```python
from build123d import *

# Parameters (mm, degrees)
SKETCH1_R           = 1.25
BOSS_EXTRUDE1_DEPTH = 1.5
SKETCH3_W           = 18.5
SKETCH3_H           = 10
BOSS_EXTRUDE2_DEPTH = 2.53


with BuildPart() as part:
    # Sketch1 → Boss-Extrude1 (new body)
    with BuildSketch(Plane(origin=(0, 0, 0), x_dir=(1, 0, 0), z_dir=(0, 1, 0))):
        with BuildLine():
            Line((31.88, 2.5), (31.88, 18.9))
            ThreePointArc((31.88, 18.9), (31.147766953, 20.667766953), (29.38, 21.4))
            Line((29.38, 21.4), (0, 21.4))
            Line((0, 21.4), (0, 0))
            Line((0, 0), (29.38, 0))
            ThreePointArc((29.38, 0), (31.147766953, 0.732233047), (31.88, 2.5))
        make_face()
        with Locations((29.38, 2.5)):
            Circle(SKETCH1_R, mode=Mode.SUBTRACT)
        with Locations((29.38, 18.9)):
            Circle(SKETCH1_R, mode=Mode.SUBTRACT)
    extrude(amount=BOSS_EXTRUDE1_DEPTH)

    # Sketch3 → Boss-Extrude2 (add)
    with BuildSketch(Plane(origin=(0, 1.5, 0), x_dir=(1, 0, 0), z_dir=(0, 1, 0))):
        with Locations((22.63, 10.7)):
            Rectangle(SKETCH3_W, SKETCH3_H)
    extrude(amount=BOSS_EXTRUDE2_DEPTH)


solid = part.part
```
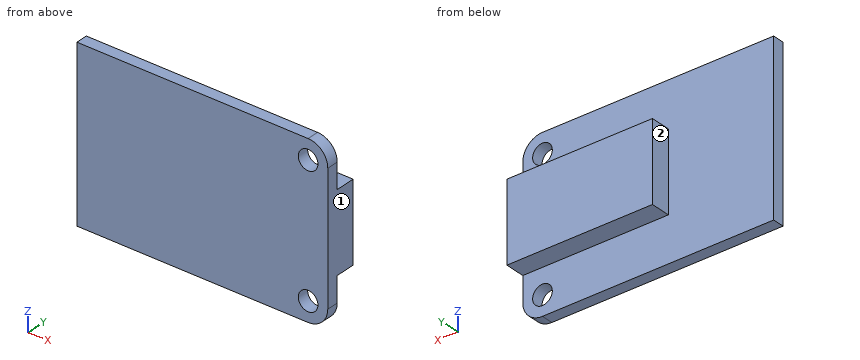
Geometry: final body of the model. Coordinates: model frame, mm. Face numbers are marked on the shaded views. A direction names the side the tool comes from. Give positions to 0.01 mm unless a question says otherwise; leave off trailing zeros. Order: outer loops, then holes, each group sorted by start corner. A loop starts at its lowest first (then second) coordinate and runs counter-clockwise, first axis right, second up. Notation, with made-up numbers: M -15.75,28.25 L -7.75,28.25 A13 ccw -7.75,50.25 Z; hole C 66,5 d4. An arc over 180 degrees is marked long. Answer as CSV lines item,"result". Start each with the question number.
1) Set-up query: the marked faces 1 and 2. Return all of +Z, -Z, +X, -X, +Y, -Y with unobstructed straight access to the full face (end or side cutting, diameter ignored); none if empty.
2) Cut plane A-A (x = 27). Output: boundary loops of the cut face in (y, z).
3) Cut plane C-C (y = 2.8). Output: boundary loops of the cut face in (x, z).
4) Cut plane D-D (x = 8). Output: boundary loops of the cut face in (y, z).
5) First-contact query: P1, Ø6, axis at x = 10, z = -10.5, coming from the -Y side; P2, Ø1.5, axis at x = 29.38, z = -18.9, coming from the +Y side. Flat tips, straight axial feed; report the tip coordinate or a pass-through.
6) Line query: line 1 (Z direction, x = 29.38, y = 1); line 2 (X direction, y = 1.05, z = -18.9); line 3 (X direction, y = 2.4, z = -14.5). Output: solid intervals per line, ascending. Write a range as from..to.
7) Cut plane B-B (z = -14.75). Output: boundary loops of the cut face in (x, y).
Findings below:
1,face 1,"+Z, -Z, +X, +Y, -Y"
1,face 2,"+Z, -Z, -X, +Y"
2,outline,"M 0,-21.4 L 1.5,-21.4 L 1.5,-15.7 L 4.03,-15.7 L 4.03,-5.7 L 1.5,-5.7 L 1.5,0 L 0,0 Z"
3,outline,"M 13.38,-15.7 L 31.88,-15.7 L 31.88,-5.7 L 13.38,-5.7 Z"
4,outline,"M 0,-21.4 L 1.5,-21.4 L 1.5,0 L 0,0 Z"
5,P1,"stops at y = 0"
5,P2,"passes through"
6,line 1,"z = -21.4..-20.15, -17.65..-3.75, -1.25..0"
6,line 2,"x = 0..28.13, 30.63..31.88"
6,line 3,"x = 13.38..31.88"
7,outline,"M 0,0 L 31.88,0 L 31.88,4.03 L 13.38,4.03 L 13.38,1.5 L 0,1.5 Z"
